Design review of the part built by this model. Coordinates are the model's own, in mm. Face numbers are marked on the shaded views. A direction names the side the tool comes from. Give positions to 0.01 mm unless a question says otherwise; leave off trailing zeros. Write each loop counter-clockwise with the first axis right and the second up, starting at its lowest first coordinate (ties: lowest second). Pieces come first, ordered by that corner, then holes. Notation, with made-up numbers: M 51,-1.75 L 69,-1.75 A14 ccw 69,3.25 Z; hole C 54,88 d9. An arc over 180 degrees is marked long. One line per item, written item: value. Start each with the question number.
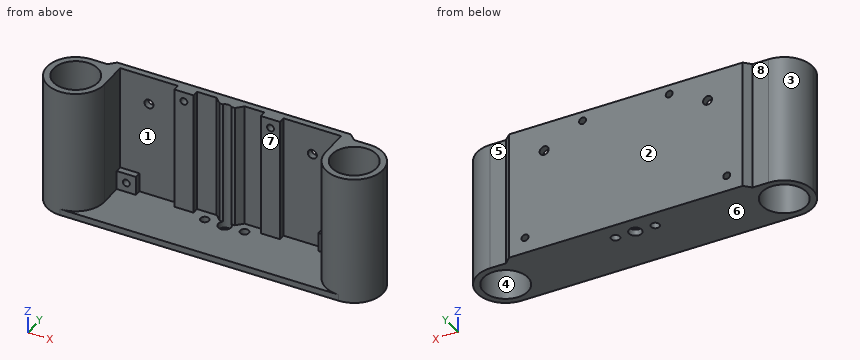
```python
from build123d import *

# Parameters (mm, degrees)
F0_R      = 11.1125
F1_DEPTH  = 65.211198
F3_DEPTH  = 3.175
F4_R      = 14.28749
F5_R      = 2.2479
F5_R_2    = 1.7272
F6_DEPTH  = 6.35
F7_R      = 3.175
F7_R_2    = 2.15265
F8_DEPTH  = 65.211198
F9_W      = 12.9742907321
F9_H      = 62.036198
F10_DEPTH = 3.175
F11_SIZE  = 3.17499


# Not quite as in the source:
# - a fillet or chamfer is up to 0.001 mm smaller than in the source, because OpenCascade refuses the exact size
# - a feature names something its author has since deleted; it is built from what else it names


with BuildPart() as f1:
    # F0 (on Top) → F1 (new body)
    with BuildSketch(Plane.XY):
        with BuildLine():
            Line((22.225, 0), (0, 0))
            Line((0, 0), (0, -14.2875))
            ThreePointArc((0, -14.2875), (14.2875, -28.575), (28.575, -14.2875))
            Line((28.575, -14.2875), (28.575, -3.175))
            Line((28.575, -3.175), (138.2559846, -3.175))
            Line((138.2559846, -3.175), (138.2559846, -14.2875))
            ThreePointArc((138.2559846, -14.2875), (152.5434846, -28.575), (166.8309846, -14.2875))
            Line((166.8309846, -14.2875), (166.8309846, 0))
            Line((166.8309846, 0), (144.6059846, 0))
            Line((144.6059846, 0), (144.6059846, 3.175))
            Line((144.6059846, 3.175), (22.225, 3.175))
            Line((22.225, 3.175), (22.225, 0))
        make_face()
        with Locations((14.2875, -14.2875)):
            Circle(F0_R, mode=Mode.SUBTRACT)
        with Locations((152.5434846, -14.2875)):
            Circle(F0_R, mode=Mode.SUBTRACT)
    extrude(amount=F1_DEPTH)

    # F2 (on face) → F3 (join)
    with BuildSketch(Plane(origin=(0, 0, 0), x_dir=(1, 0, 0), z_dir=(0, 0, -1))):
        with BuildLine():
            Line((152.5434846, 28.575), (14.2875, 28.575))
            ThreePointArc((14.2875, 28.575), (24.3902881362, 24.3902881362), (28.575, 14.2875))
            Line((28.575, 14.2875), (28.575, 3.175))
            Line((28.575, 3.175), (138.2559846, 3.175))
            Line((138.2559846, 3.175), (138.2559846, 14.2875))
            ThreePointArc((138.2559846, 14.2875), (142.4406964638, 24.3902881362), (152.5434846, 28.575))
        make_face()
    extrude(amount=-F3_DEPTH)

    # F4 (radius 14.2875 in the source; OpenCascade refuses exactly that, so slightly less here)
    f4_edges = [f1.edges().sort_by_distance(p)[0] for p in [
        (0, 0, 32.605599),
        (166.830985, 0, 32.605599),
    ]]
    fillet(f4_edges, radius=F4_R)

    # F5 (on face) → F6 (cut, through all)
    with BuildSketch(Plane(origin=(0, 3.175, 0), x_dir=(-1, 0, 0), z_dir=(0, 1, 0))):
        with Locations((-123.9684846, 50.923698)):
            Circle(F5_R)
        with Locations((-104.9184846, 60.448698)):
            Circle(F5_R_2)
        with Locations((-61.9125, 60.448698)):
            Circle(F5_R_2)
        with Locations((-42.8625, 50.923698)):
            Circle(F5_R)
        with Locations((-133.4934846, 7.9375)):
            Circle(F5_R_2)
        with Locations((-33.3375, 7.9375)):
            Circle(F5_R_2)
    extrude(amount=-F6_DEPTH, mode=Mode.SUBTRACT)

    # F7 (on face) → F8 (cut, through all)
    with BuildSketch(Plane(origin=(0, 0, 0), x_dir=(1, 0, 0), z_dir=(0, 0, -1))):
        with Locations((83.4154923, 5.4845204)):
            Circle(F7_R)
        with Locations((73.5203484069, 5.4845204)):
            Circle(F7_R_2)
        with Locations((93.3106361931, 5.4845204)):
            Circle(F7_R_2)
    extrude(amount=-F8_DEPTH, mode=Mode.SUBTRACT)

    # F9 (on face) → F10 (cut)
    with BuildSketch(Plane.XZ.offset(3.175)):
        Polygon((57.15, 65.211198), (28.575, 65.211198), (28.575, 12.7), (38.1, 12.7), (38.1, 3.175), (57.15, 3.175), align=None)
        Polygon((138.2559846, 12.7), (138.2559846, 65.211198), (109.6809846, 65.211198), (109.6809846, 3.175), (128.7309846, 3.175), (128.7309846, 12.7), align=None)
        with Locations((73.162145366, 34.193099)):
            Rectangle(F9_W, F9_H)
        with Locations((93.668839234, 34.193099)):
            Rectangle(F9_W, F9_H)
    extrude(amount=-F10_DEPTH, mode=Mode.SUBTRACT)

    # F11 (size 3.175 in the source; OpenCascade refuses exactly that, so slightly less here)
    f11_edges = [f1.edges().sort_by_distance(p)[0] for p in [
        (22.225, 3.175, 32.605599),
        (144.605985, 3.175, 32.605599),
        (87.181694, 0, 34.193099),
        (79.649291, 0, 34.193099),
    ]]
    chamfer(f11_edges, length=F11_SIZE)


solid = f1.part
```
Q1. Wall thickness on line 1 (X direction, y = -20, z = 38); line 2 (X direction, y = -13, z = 30) (3 decimals); line 3 (X direction, y = 2, z = 51): over which ranges is each line inside the solid? List them lowest first. Write a range as from..to.
Q2. Take a section at C-C, the plane x = 55.5. Give the boundary of the cut face in (y, z) (3 decimals), then the cut area to 3 significant figures.
Q3. Take a section at B-B, the plane y = -11. Give the boundary of the cut face in (x, z) (3 decimals).
Q4. The part is to be moulded in two halves that separate along X. For the marked faces 1, 2 and 3, say which applies: pulls with the +X half, pulls with the -X half, needs draft (parallel to the pull), parting line crosses it, or undercut.
Q5. Machinability: for the marked faces 4, 5, 6, 7 and 8, which of the approach directions +Z, -Z, +X, -X, +Y, -Y give a long, thin tool a straight path to every point of the face, cutting with its end or side? Answer none if there is none.
Q6. For P1, Ø3.5, axis at y = -1.5, z = 27, coming from the -X side; P2, Ø8, axis at x = 72.5, z = 44, coming from the -Y side; P3, Ø5, axis at x = 35.5, z = 6, coming from the -Y side (3 decimals), all flat-tipped, find the tip position at first contact; note any pin that passes through.
Q7. Take a section at D-D, the plane y = -17.5. Give the boundary of the cut face in (x, z) (1 decimal), then the cut area to 3 significant figures.
Q8. Take a section at A-A, the plane z = 19. State how many separate pieces and enclosed holes the cut face has, then the cut area to 3 significant figures.
Results list:
1. line 1: x = 1.19..4.76, 23.82..27.38, 139.45..143.01, 162.08..165.64
1. line 2: x = 0.058..3.25, 25.325..28.575, 138.256..141.506, 163.581..166.773
1. line 3: x = 24.22..40.62, 45.11..121.72, 126.22..142.61
2. outline: M -28.575,0 L 3.175,0 L 3.175,65.211 L 0,65.211 L 0,3.175 L -28.575,3.175 Z
2. area: 298 mm^2
3. outline: M 0.383,0 L 3.672,0 L 3.672,65.211 L 0.383,65.211 Z; M 24.903,0 L 141.928,0 L 141.928,65.211 L 138.256,65.211 L 138.256,3.175 L 28.575,3.175 L 28.575,65.211 L 24.903,65.211 Z; M 163.159,0 L 166.448,0 L 166.448,65.211 L 163.159,65.211 Z
4. face 1: undercut
4. face 2: needs draft
4. face 3: pulls with the -X half
5. face 4: +Z, -Z
5. face 5: +Z, -Z, +X, +Y
5. face 6: -Z, +X, -X, +Y, -Y
5. face 7: +Z, -Y
5. face 8: +Z, -Z, -X, +Y
6. P1: stops at x = 5.22
6. P2: stops at y = -0.03
6. P3: stops at y = -3.175
7. outline: M 0.4,0 L 3.6,0 L 3.6,65.2 L 0.4,65.2 Z; M 24.9,0 L 141.9,0 L 141.9,65.2 L 138.6,65.2 L 138.6,3.2 L 28.2,3.2 L 28.2,65.2 L 24.9,65.2 Z; M 163.2,0 L 166.5,0 L 166.5,65.2 L 163.2,65.2 Z
7. area: 1,210 mm^2
8. separate pieces: 1
8. enclosed holes: 2
8. area: 1,060 mm^2
